from build123d import *

# Parameters (mm, degrees)
SKETCH_1_W      = 55
SKETCH_1_H      = 15
SKETCH_1_R      = 2.6
EXTRUDE_1_DEPTH = 3


with BuildPart() as part:
    # Эскиз1 → Бобышка-Вытянуть1 (new body)
    with BuildSketch(Plane(origin=(0, 0, 0), x_dir=(1, 0, 0), z_dir=(0, 1, 0))):
        Rectangle(SKETCH_1_W, SKETCH_1_H)
        Circle(SKETCH_1_R, mode=Mode.SUBTRACT)
        with Locations((20, 0)):
            Circle(SKETCH_1_R, mode=Mode.SUBTRACT)
        with Locations((-20, 0)):
            Circle(SKETCH_1_R, mode=Mode.SUBTRACT)
    extrude(amount=EXTRUDE_1_DEPTH)


solid = part.part
The model under review builds one solid part; all positions refer to its coordinate system, in mm. Coordinates: 2 decimals unless noted, no trailing zeros. Loops run counter-clockwise (first coordinate to the right, second up) from the corner with the lowest first, then second, coordinate; pieces in that order, holes last. Notation, with made-up numbers: M 9,52.25 L 39,52.25 A11 cw 39,59.25 Z; hole C -35.5,-38 d6. An arc over 180 degrees is marked long. Put each result on its own line as item: value. Start each with the question number.
Q1. Add section D-D (x = 22). Write out the cut boundary in (y, z).
Q2. Add section A-A (z = 0). Write out the cut boundary in (x, y), and give its area (3 significant figures).
Q3. The part is to be moulded in two halves that separate along Z. For faces 1 (the flat face through (0, 1, -7.5)), 2 (the cylindrical face through (-0.338, 1.479, -2.578)), 3 (the flat face through (27.5, 1, 0)), say which applies: +Z half, -Z half, draft (parallel to the pull), parting line (faces both ways), or undercut.
Q4. Add section C-C (y = 2.3). Write out the cut boundary in (x, z).
Q5. Wall thickness on line 1 (X direction, y = 2, z = 0); line 2 (Z direction, x = -20, y = 2.3); line 3 (X direction, y = 2, z = -1.75): over which ranges is each line inside the solid? List them lowest first.
Q6. Add section B-B (x = 0). Write out the cut boundary in (y, z).
Answers:
1. outline: M 0,-7.5 L 3,-7.5 L 3,-1.66 L 0,-1.66 Z; M 0,1.66 L 3,1.66 L 3,7.5 L 0,7.5 Z
2. outline: M -27.5,0 L -22.6,0 L -22.6,3 L -27.5,3 Z; M -17.4,0 L -2.6,0 L -2.6,3 L -17.4,3 Z; M 2.6,0 L 17.4,0 L 17.4,3 L 2.6,3 Z; M 22.6,0 L 27.5,0 L 27.5,3 L 22.6,3 Z
2. area: 118 mm^2
3. face 1: -Z half
3. face 2: undercut
3. face 3: draft
4. outline: M -27.5,-7.5 L 27.5,-7.5 L 27.5,7.5 L -27.5,7.5 Z; hole C -20,0 d5.2; hole C 0,0 d5.2; hole C 20,0 d5.2
5. line 1: x = -27.5 to -22.6, -17.4 to -2.6, 2.6 to 17.4, 22.6 to 27.5
5. line 2: z = -7.5 to -2.6, 2.6 to 7.5
5. line 3: x = -27.5 to -21.92, -18.08 to -1.92, 1.92 to 18.08, 21.92 to 27.5
6. outline: M 0,-7.5 L 3,-7.5 L 3,-2.6 L 0,-2.6 Z; M 0,2.6 L 3,2.6 L 3,7.5 L 0,7.5 Z
